Source: CAD feature listing. Evaluate the final solid. Frame: model axes, mm. A direction names the side the tool comes from. Coordinates: 2 decimals unless noted, no trailing zeros. Order: outer loops, then holes, each group sorted by start corner. A loop starts at its lowest first (then second) coordinate and runs counter-clockwise, first axis right, second up.
```python
from build123d import *

# Parameters (mm, degrees)
SKETCH1_W           = 145
SKETCH1_H           = 20
SKETCH1_R           = 2.75
BOSS_EXTRUDE1_DEPTH = 2


with BuildPart() as part:
    # Sketch1 → Boss-Extrude1 (new body)
    with BuildSketch(Plane.XY):
        Rectangle(SKETCH1_W, SKETCH1_H)
        with Locations((62.5, 0)):
            Circle(SKETCH1_R, mode=Mode.SUBTRACT)
        with Locations((42.5, 0)):
            Circle(SKETCH1_R, mode=Mode.SUBTRACT)
        with BuildLine():
            Line((-68, -3), (-68, 3))
            ThreePointArc((-68, 3), (-65, 6), (-62, 3))
            Line((-62, 3), (-62, -3))
            ThreePointArc((-62, -3), (-65, -6), (-68, -3))
        make_face(mode=Mode.SUBTRACT)
        with BuildLine():
            Line((-48, -3), (-48, 3))
            ThreePointArc((-48, 3), (-45, 6), (-42, 3))
            Line((-42, 3), (-42, -3))
            ThreePointArc((-42, -3), (-45, -6), (-48, -3))
        make_face(mode=Mode.SUBTRACT)
    extrude(amount=BOSS_EXTRUDE1_DEPTH)


solid = part.part
```
Q1. Section query C-C on z = 1.2. Output: boundary loops of the cut face in (x, y).
Solutions:
outline: (-72.5, -10) - (72.5, -10) - (72.5, 10) - (-72.5, 10) - close; hole (-68, -3) arc R3 ccw to (-62, -3) - (-62, 3) arc R3 ccw to (-68, 3) - close; hole (-48, -3) arc R3 ccw to (-42, -3) - (-42, 3) arc R3 ccw to (-48, 3) - close; hole circle Ø5.5 at (42.5, 0); hole circle Ø5.5 at (62.5, 0)
Q2. Pull-direction query (Y, two-part tool) for faces 1 (the cylindrical face through (-65, -6, 1)), 2 (the cylindrical face through (-65, 6, 1)), 3 (the flat face through (-1, 0, 0)); classes: pulls with the +Y half, pulls with the -Y half, needs draft (parallel to the pull), parting line crosses it, or undercut.
Solutions:
face 1: undercut
face 2: undercut
face 3: needs draft
Q3. Section query A-A on x = 42.5. Output: boundary loops of the cut face in (y, z), plus the area to 3 significant figures.
Solutions:
outline: (-10, 0) - (-2.75, 0) - (-2.75, 2) - (-10, 2) - close; (2.75, 0) - (10, 0) - (10, 2) - (2.75, 2) - close
area: 29.0 mm2
Q4. Set-up query: faces 4 (the flat face through (-1, 0, 2)), 5 (the cylindrical face through (-45, -6, 1)). Return all of +Z, -Z, +X, -X, +Y, -Y with unobstructed straight access to the full face (end or side cutting, diameter ignored); none if empty.
Solutions:
face 4: +Z, +X, -X, +Y, -Y
face 5: +Z, -Z
Q5. Section query D-D on x = -45. Output: boundary loops of the cut face in (y, z).
Solutions:
outline: (-10, 0) - (-6, 0) - (-6, 2) - (-10, 2) - close; (6, 0) - (10, 0) - (10, 2) - (6, 2) - close
Q6. Material intervals for line 1 along X through (y, z) = (4.5, 0.75); line 2 along X through (y, z) = (-2, 0.9); line 3 along Y through (x, z) = (62.5, 0.5), sorted ascending.
Solutions:
line 1: x = -72.5 to -67.6, -62.4 to -47.6, -42.4 to 72.5
line 2: x = -72.5 to -68, -62 to -48, -42 to 40.61, 44.39 to 60.61, 64.39 to 72.5
line 3: y = -10 to -2.75, 2.75 to 10
Q7. Section query B-B on y = 0. Output: boundary loops of the cut face in (x, z), plus the area to 3 significant figures.
Solutions:
outline: (-72.5, 0) - (-68, 0) - (-68, 2) - (-72.5, 2) - close; (-62, 0) - (-48, 0) - (-48, 2) - (-62, 2) - close; (-42, 0) - (39.75, 0) - (39.75, 2) - (-42, 2) - close; (45.25, 0) - (59.75, 0) - (59.75, 2) - (45.25, 2) - close; (65.25, 0) - (72.5, 0) - (72.5, 2) - (65.25, 2) - close
area: 244 mm2
